from build123d import *

# Parameters (mm, degrees)
BOSS_EXTRU_1_DEPTH      = 3
ESQUISSE2_R             = 1.5
ENL_V_MAT_EXTRU_1_DEPTH = 48.265209192
BOSS_EXTRU_2_DEPTH      = 3
CONG_1_R                = 20
ESQUISSE4_R             = 2
ENL_V_MAT_EXTRU_2_DEPTH = 56.901699437
CONG_3_R                = 2


with BuildPart() as part:
    # Esquisse1 → Boss.-Extru.1 (new body)
    with BuildSketch(Plane.XY):
        with BuildLine():
            Line((-27.5, 0), (27.5, 0))
            ThreePointArc((27.5, 0), (40, -12.5), (27.5, -25))
            Line((27.5, -25), (-27.5, -25))
            ThreePointArc((-27.5, -25), (-40, -12.5), (-27.5, 0))
        make_face()
    extrude(amount=BOSS_EXTRU_1_DEPTH)

    # Esquisse2 → Enlèv. mat.-Extru.1 (cut, through all)
    with BuildSketch(Plane.XY.offset(3)):
        with Locations((-22.5, -12.5)):
            Circle(ESQUISSE2_R)
        with Locations((22.5, -12.5)):
            Circle(ESQUISSE2_R)
    extrude(amount=-ENL_V_MAT_EXTRU_1_DEPTH, mode=Mode.SUBTRACT)

    # Esquisse3 → Boss.-Extru.2 (add)
    with BuildSketch(Plane.XZ.offset(25)):
        with BuildLine():
            Line((-12.5, 0), (12.5, 0))
            Line((12.5, 0), (12.5, 27))
            ThreePointArc((12.5, 27), (11.621320344, 29.121320344), (9.5, 30))
            Line((9.5, 30), (-9.5, 30))
            ThreePointArc((-9.5, 30), (-11.621320344, 29.121320344), (-12.5, 27))
            Line((-12.5, 27), (-12.5, 0))
        make_face()
    extrude(amount=BOSS_EXTRU_2_DEPTH)

    # Congé1
    # the kernel refuses this fillet: 20 mm, written as the material it adds along each edge
    with BuildSketch(Plane(origin=(12.5, -25, 0), x_dir=(1, 0, 0), z_dir=(0, 0, 1)), Plane(origin=(-12.5, -25, 3), x_dir=(-1, 0, 0), z_dir=(0, 0, -1))) as cong_1_piece_1:
        with BuildLine():
            CenterArc((10.535653753, -20), CONG_1_R, 90, 31.788330617)
            Line((0, -3), (0, 0))
            Line((0, 0), (10.535653753, 0))
        make_face()
    extrude(amount=3)

    # Esquisse4 → Enlèv. mat.-Extru.2 (cut, through all)
    with BuildSketch(Plane(origin=(0, -25, 0), x_dir=(1, 0, 0), z_dir=(0, 1, 0))):
        with Locations(Location((0, -20, 0), (0, 0, 270))):
            Circle(ESQUISSE4_R)
    extrude(amount=-ENL_V_MAT_EXTRU_2_DEPTH, mode=Mode.SUBTRACT)

    # Congé3
    cong_3_edges = [part.edges().sort_by_distance(p)[0] for p in [
        (-12.5, -25, 15),
        (12.5, -25, 15),
        (11.621320344, -25, 29.121320344),
        (0, -25, 30),
        (-11.621320344, -25, 29.121320344),
    ]]
    fillet(cong_3_edges, radius=CONG_3_R)


solid = part.part
Verification items for the finished model (mm, model axes). A direction names the side the tool comes from. Coordinates: 2 decimals unless noted, no trailing zeros. Order: outer loops, then holes, each group sorted by start corner. A loop starts at its lowest first (then second) coordinate and runs counter-clockwise, first axis right, second up. Notation, with made-up numbers: M 88,40 L 126,40 A19 cw 126,53 Z; hole C -26,32.5 d6. An arc over 180 degrees is marked long. One line per item, written item: value. Start each with the question number.
Item 1: Thickness scan on probe 1 along Y at (x, z) = (22.5, 2.15); probe 2 along X at (y, z) = (-27.05, 20); probe 3 along Y at (x, z) = (7.5, 9.25). Record the ranges inside material, lowest first.
Item 2: Access from +Z, -Z, +X, -X, +Y, -Y to the whole of each face (thin tool, end or side, straight path). Record for faces 4 (the cylindrical face through (11.93, -25.6, 15.17)), 5 (the flat face through (-25, -25, 1)), 6 (the flat face through (0, -25, 16)), 7 (the flat face through (25, -25, 1)).
Item 3: Sectioned sample at A-A on x = 0. Record the cut outline in (y, z), then the cut area to 3 significant figures.
Item 4: Depth check by flat-ended pin: P1, Ø6, axis at x = -6.5, y = -23, coming from the +Z side; P2, Ø2.5, axis at x = 24.5, z = 1.5, coming from the -Y side; P3, Ø0.5, axis at y = -27.5, z = 16, coming from the -X side. Enter the tip coordinate at first touch or a pass-through.
Item 5: Mould release check, pull along X, two halves, no side actions. Record for faces 1 (the cylindrical face through (39.997, -12.225, 1.479)), 2 (the cylindrical face through (-39.997, -12.775, 1.479)), 3 (the cylindrical face through (-24, -12.43, 1.52)): pulls with the +X half, pulls with the -X half, needs draft (parallel to the pull), parting line crosses it, or undercut.
Item 6: Sectioned sample at B-B on y = -12.5. Record the cut outline in (x, z), then the cut area to 3 significant figures.
Item 7: Sectioned sample at D-D on z = 14. Record the cut outline in (x, y).
Item 8: Sectioned sample at C-C on z = 20. Record the cut outline in (x, y).
Calculated:
1. probe 1: -25.01 to -14, -11 to 0
1. probe 2: -12.5 to -2, 2 to 12.5
1. probe 3: -28 to -25
2. face 4: +Z, +X, +Y
2. face 5: +Z, -Z, -X, -Y
2. face 6: +Z, +X, -X, +Y
2. face 7: +Z, -Z, +X, -Y
3. outline: M -28,0 L 0,0 L 0,3 L -25,3 L -25,18 L -28,18 Z; M -28,22 L -25,22 L -25,28 A2 ccw -27,30 L -28,30 Z
3. area: 152 mm^2
4. P1: z = 29.73
4. P2: y = -25
4. P3: x = -12.5
5. face 1: pulls with the +X half
5. face 2: pulls with the -X half
5. face 3: undercut
6. outline: M -40,0 L -24,0 L -24,3 L -40,3 Z; M -21,0 L 21,0 L 21,3 L -21,3 Z; M 24,0 L 40,0 L 40,3 L 24,3 Z
6. area: 222 mm^2
7. outline: M -12.5,-28 L 12.5,-28 L 12.5,-27 A2 ccw 10.5,-25 L -10.5,-25 A2 ccw -12.5,-27 Z
8. outline: M -12.5,-28 L -2,-28 L -2,-25 L -10.5,-25 A2 ccw -12.5,-27 Z; M 2,-28 L 12.5,-28 L 12.5,-27 A2 ccw 10.5,-25 L 2,-25 Z
